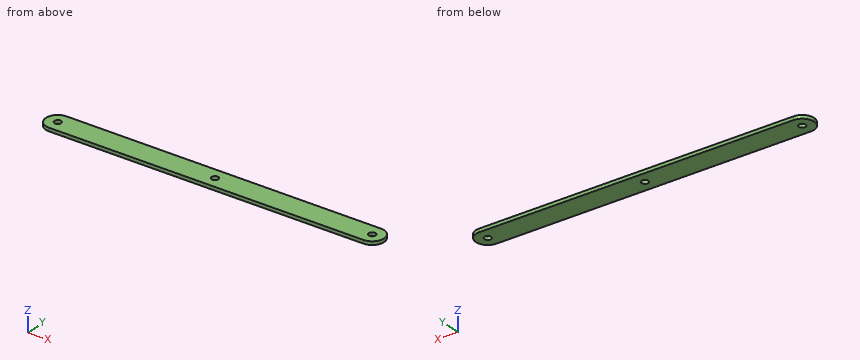
from build123d import *

# Parameters (mm, degrees)
SKETCH1_W           = 500
SKETCH1_H           = 35
BOSS_EXTRUDE1_DEPTH = 2.5
FILLET1_R           = 17.5
SKETCH2_R           = 5
CUT_EXTRUDE1_DEPTH  = 5


with BuildPart() as part:
    # Sketch1 → Boss-Extrude1 (new, symmetric)
    with BuildSketch(Plane.XY):
        Rectangle(SKETCH1_W, SKETCH1_H)
    extrude(amount=BOSS_EXTRUDE1_DEPTH, both=True)

    # Fillet1
    fillet1_edges = [part.edges().sort_by_distance(p)[0] for p in [
        (-250, -17.5, 0),
        (-250, 17.5, 0),
        (250, -17.5, 0),
        (250, 17.5, 0),
    ]]
    fillet(fillet1_edges, radius=FILLET1_R - 0.0001)  # a hair under: the kernel refuses the full size

    # Sketch2 → Cut-Extrude1 (cut)
    with BuildSketch(Plane.XY.offset(2.5)):
        Circle(SKETCH2_R)
        with Locations((232.5, 0)):
            Circle(SKETCH2_R)
        with Locations(Location((-232.5, 0, 0), (0, 0, 180))):
            Circle(SKETCH2_R)
    extrude(amount=-CUT_EXTRUDE1_DEPTH, mode=Mode.SUBTRACT)


solid = part.part
Geometry: final body of the model. Coordinates: model frame, mm. Give positions to 0.01 mm unless a question says otherwise; leave off trailing zeros. Order: outer loops, then holes, each group sorted by start corner. A loop starts at its lowest first (then second) coordinate and runs counter-clockwise, first axis right, second up. Notation, with made-up numbers: (7, -4) -> (30, -4) arc R26 ccw to (30, 24) -> close; hole circle Ø4 at (-21, 20). An arc over 180 degrees is marked (long way). Answer as a JSON object with one key per item and string values.
Q1. First-contact query: pin 1 (9 mm diameter, centred on x = 0, y = 0, fed in from +Z); pin 2 (11.5 mm diameter, centred on x = 232.5, y = 0, fed in from +Z); pin 3 (1 mm diameter, centred on y = 3, z = 1.5, fed in from -X); pin 4 (1 mm diameter, centred on y = 12.5, z = -1, fed in from -X). Flat tips, straight axial feed; report the tip coordinate or a pass-through.
Entries:
{"pin 1": "passes through", "pin 2": "stops at z = 2.5", "pin 3": "stops at x = -249.82", "pin 4": "stops at x = -245.24"}
Q2. Section A-A (z = 0.75). State how many separate pieces and enclosed holes the cut face has, plus the area to 3 significant figures.
Entries:
{"separate pieces": "1", "enclosed holes": "3", "area": "17,000 mm^2"}
Q3. Section B-B (x = 0). Output: boundary loops of the cut face in (y, z), plus the area to 3 significant figures.
Entries:
{"outline": "(-17.5, -2.5) -> (-5, -2.5) -> (-5, 2.5) -> (-17.5, 2.5) -> close; (5, -2.5) -> (17.5, -2.5) -> (17.5, 2.5) -> (5, 2.5) -> close", "area": "125 mm^2"}
Q4. Material intervals for probe 1 along Y at (x, z) = (0, 0.65); probe 2 along X at (y, z) = (-13.5, -0.7); probe 3 along X at (y, z) = (-6.5, 0.4), sorted ascending.
Entries:
{"probe 1": "y = -17.5 to -5, 5 to 17.5", "probe 2": "x = -243.64 to 243.64", "probe 3": "x = -248.75 to 248.75"}
